Autodesk Fusion 360 part; units mm, degrees
sketch " Compartment Divet" plane through (0, 0, 0) normal (0, 0, 1) x (1, 0, 0)
  line L0 (5, 5) -> (25, 5) construction
  line L1 (25, 5) -> (25, 35) construction
  line L2 (25, 35) -> (5, 35) construction
  line L3 (5, 35) -> (5, 5) construction
  line L4 (5, 35) -> (25, 35)
  line L5 (25, 35) -> (25, 5)
  line L6 (25, 5) -> (5, 5)
  line L7 (5, 5) -> (5, 35)
  dimension "d3" = 20
  dimension "d4" = 30
sketch "Compartment Body" plane through (0, 0, 0) normal (0, 0, 1) x (1, 0, 0)
  line L0 (0, 0) -> (30, 0)
  line L1 (30, 0) -> (30, 100)
  line L2 (30, 100) -> (0, 100)
  line L3 (0, 100) -> (0, 0)
  line L4 (5, 95) -> (25, 95)
  line L5 (25, 95) -> (25, 5)
  line L6 (25, 5) -> (5, 5)
  line L7 (5, 5) -> (5, 95)
  line L8 (5, 95) -> (25, 95)
  line L9 (25, 95) -> (25, 77)
  line L10 (25, 77) -> (5, 77)
  line L11 (5, 77) -> (5, 95)
  line L12 (5, 71) -> (25, 71)
  line L13 (25, 71) -> (25, 53)
  line L14 (25, 53) -> (5, 53)
  line L15 (5, 53) -> (5, 71)
  line L16 (5, 47) -> (25, 47)
  line L17 (25, 47) -> (25, 29)
  line L18 (25, 29) -> (5, 29)
  line L19 (5, 29) -> (5, 47)
  line L20 (5, 23) -> (25, 23)
  line L21 (25, 23) -> (25, 5)
  line L22 (25, 5) -> (5, 5)
  line L23 (5, 5) -> (5, 23)
  dimension "d7" = 30
  dimension "d8" = 100
  dimension "d11" = 18
  dimension "d12" = 18
  dimension "d13" = 18
  dimension "d14" = 18
extrude "Extrude2" add sketch " Compartment Divet" against normal blind 10 makes body 1
extrude "Extrude3" add sketch "Compartment Body" along normal blind 5 contours L4 L5 L7 L8 L9 L10 L11 | L5 L7 L12 L13 L14 L15 | L5 L7 L16 L17 L18 L19 | L5 L6 L7 L20 L21 L22 L23 bodies 1 makes body 2 at (11.6667, 65, 0) makes body 3 at (11.6667, 89, 0)
extrude "Extrude4" add sketch "Compartment Body" along normal blind 10 contours L0 L1 L2 L3 | L5 L7 L10 L12 | L5 L7 L14 L16 | L5 L7 L18 L20 bodies 1 2 3
extrude "Extrude5" cut 4 faces at (11.6667, 17, 5) (18.3333, 41, 5) (11.6667, 65, 5) (11.6667, 89, 5) along direction (0, 0, -1) blind 3 on bodies 1 bodies 1
Check sheet for the modelled part. Datum: model origin and axes. Units: mm. A direction names the side the tool comes from. Round coordinates to 2 decimals unless told otherwise and drop trailing zeros. Order: outer loops, then holes, each group sorted by start corner. A loop starts at its lowest first (then second) coordinate and runs counter-clockwise, first axis right, second up.
1) Tool access check on faces 5 (the flat face through (5, 20, -5)), 6 (the flat face through (15, 35, -5)), 7 (the flat face through (15, 71, 6)), 8 (the flat face through (15, 20, -10)), 9 (the flat face through (25, 20, -5)). Record the directions out of +Z, -Z, +X, -X, +Y, -Y that give a thin tool (end or side, any length) a straight path to the whole face; none if there is none.
2) Section check C-C (z = -4.25). Record the boundary of the cut face in (x, y).
3) Go/stop test with flat-tipped pins: pin 1 Ø14.5 at (x, y) = (17, 37.5) entering from +Z; pin 2 Ø3 at (x, z) = (17.5, -6) entering from -Y; pin 3 Ø3 at (x, y) = (19.5, 62.5) entering from -Z. Record where each tip stops, or that it passes through.
4) Section check B-B (y = 13.5). Record the boundary of the cut face in (x, z), and give its area (3 significant figures).
5) Section check D-D (y = 64.5). Record the boundary of the cut face in (x, z), and give its area (3 significant figures).
6) Mould release check, pull along Y, two halves, no side actions. Record for faces 1 (the flat face through (15, 0, 5)), 2 (the flat face through (30, 49, 5)), 3 (the flat face through (15, 53, 6)), 4 (the flat face through (25, 14, 6)): +Y half, -Y half, draft (parallel to the pull), parting line (faces both ways), or undercut.
7) Section check A-A (x = 10.5). Record the boundary of the cut face in (y, z), and give its area (3 significant figures).
8) Scan lines: line 1 (Y direction, x = 16.25, z = 3.75); line 2 (X direction, y = 92, z = 6); line 3 (X direction, y = 20.5, z = -2). Record each from-to range of solid material in increasing order.
Result:
1. face 5: -Z, -X, +Y, -Y
1. face 6: -Z, +X, -X, +Y
1. face 7: +Z
1. face 8: -Z, +X, -X, +Y, -Y
1. face 9: -Z, +X, +Y, -Y
2. outline: (5, 5) - (25, 5) - (25, 35) - (5, 35) - close
3. pin 1: stops at z = 2
3. pin 2: stops at y = 5
3. pin 3: stops at z = 0
4. outline: (0, 0) - (5, 0) - (5, -10) - (25, -10) - (25, 0) - (30, 0) - (30, 10) - (25, 10) - (25, 2) - (5, 2) - (5, 10) - (0, 10) - close
4. area: 340 mm2
5. outline: (0, 0) - (30, 0) - (30, 10) - (25, 10) - (25, 2) - (5, 2) - (5, 10) - (0, 10) - close
5. area: 140 mm2
6. face 1: -Y half
6. face 2: draft
6. face 3: undercut
6. face 4: undercut
7. outline: (0, 0) - (5, 0) - (5, -10) - (35, -10) - (35, 0) - (100, 0) - (100, 10) - (95, 10) - (95, 2) - (77, 2) - (77, 10) - (71, 10) - (71, 2) - (53, 2) - (53, 10) - (47, 10) - (47, 2) - (29, 2) - (29, 10) - (23, 10) - (23, 2) - (5, 2) - (5, 10) - (0, 10) - close
7. area: 724 mm2
8. line 1: y = 0 to 5, 23 to 29, 47 to 53, 71 to 77, 95 to 100
8. line 2: x = 0 to 5, 25 to 30
8. line 3: x = 5 to 25
